Can you work these out from the model? Positions are in its coordinate system, mm. A direction names the side the tool comes from. Round coordinates to 2 decimals unless told otherwise and drop trailing zeros. Write each loop counter-clockwise with the first axis right and the second up, starting at its lowest first coordinate (ties: lowest second). Pieces come first, ordered by that corner, then holes. Notation, with made-up numbers: M -33,71 L 8,71 A22 cw 8,77 Z; hole C 38,-18 d1. An arc over 180 degrees is marked long. Answer in a Markdown table with one row per item. Add a question column.
(1) For faces 1 (the face through (76.2, -7, 9)), 2 (the face through (-76.2, -174, 85)), 3 (the face through (76.2, -151, -6)), 4 (the face through (-76.2, -7, 9)), which set-ups out of +Z, -Z, +X, -X, +Y, -Y let a thin tool reach every point of the face, with its end or its side?
(2) Suppose I cut it at D-D, the plane y = -191. Write out the boundary of the cut face in (x, z), then the cut area to 3 significant figures.
(3) Suppose I cut it at A-A, the plane z = 86.5. Write out the boundary of the cut face in (x, y).
(4) Suppose I cut it at C-C, the plane y = -152.5. Write out the boundary of the cut face in (x, z), then the cut area to 3 significant figures.
(5) If we mould it in two halves opening along X, with no side actions, what happens to faces 5 (the face through (-82.55, -174, 65)), 6 (the face through (76.2, -174, 85)), 7 (the face through (79, -50.8, 13)), 8 (the face through (64.74, 65.34, 9.66))? For each: released by +X, released by -X, zero draft, split by the parting line, or undercut.
(6) If I drill on probe 1 along Y at (x, z) = (0, 4.5); probe 2 along X at (y, z) = (-227.5, 41.5); probe 3 along Z at (x, y) = (-47, -205), over which ranges is the centre line in solid material (lowest first)?
(7) Suppose I cut it at B-B, the plane x = 0. Write out the boundary of the cut face in (y, z).
(8) I'm going to push flat-ended pins straight in: pin 1 (6 mm diameter, centred on x = 5, y = -165, fed in from +Z); pin 2 (9.5 mm diameter, centred on y = 6.5, z = 14, fed in from +X); pin 3 (9.5 mm diameter, centred on y = 5, z = 9, fed in from -X). Where does each tip first touch, or does it pass through?
from build123d import *

# Parameters (mm, degrees)
SKETCH2_W           = 152.4
SKETCH2_H           = 330.2
BOSS_EXTRUDE1_DEPTH = 19.05
SKETCH5_R           = 25.4
CUT_EXTRUDE1_DEPTH  = 266.867151976
FILLET1_R           = 38.1
BOSS_EXTRUDE2_DEPTH = 6.35


with BuildPart() as part:
    # Sketch2 → Boss-Extrude1 (new body)
    with BuildSketch(Plane.XY):
        with Locations((0, -88.9)):
            Rectangle(SKETCH2_W, SKETCH2_H)
    extrude(amount=BOSS_EXTRUDE1_DEPTH)

    # Sketch5 → Cut-Extrude1 (cut, through all)
    with BuildSketch(Plane.XY):
        with Locations(Location((0, 0, 0), (0, 0, 180))):
            Circle(SKETCH5_R)
    extrude(amount=CUT_EXTRUDE1_DEPTH, mode=Mode.SUBTRACT)

    # Fillet1
    fillet1_edges = [part.edges().sort_by_distance(p)[0] for p in [
        (-76.2, 76.2, 9.525),
        (76.2, 76.2, 9.525),
    ]]
    fillet(fillet1_edges, radius=FILLET1_R)

    # Sketch3 → Boss-Extrude2 (add)
    with BuildSketch(Plane(origin=(76.2, 0, 0), x_dir=(0, 0, -1), z_dir=(1, 0, 0))):
        Polygon((12.7, -50.8), (12.7, -254), (-190.5, -254), (-190.5, -203.2), (-38.1, -50.8), align=None)
    boss_extrude2 = extrude(amount=BOSS_EXTRUDE2_DEPTH)

    # Mirror1: Boss-Extrude2 across plane
    add(boss_extrude2.mirror(Plane(origin=(0, 0, 0), x_dir=(0, 0, 1), z_dir=(1, 0, 0))))


solid = part.part
Calculated:
| question | item | result |
|---|---|---|
| 1 | face 1 | +Z, -Z, +X, +Y |
| 1 | face 2 | +Z, +Y, -Y |
| 1 | face 3 | -Z, +Y, -Y |
| 1 | face 4 | +Z, -Z, -X, +Y |
| 2 | outline | M -82.55,-12.7 L -76.2,-12.7 L -76.2,0 L 76.2,0 L 76.2,-12.7 L 82.55,-12.7 L 82.55,178.3 L 76.2,178.3 L 76.2,19.05 L -76.2,19.05 L -76.2,178.3 L -82.55,178.3 Z |
| 2 | area | 5,330 mm² |
| 3 | outline | M -82.55,-254 L -76.2,-254 L -76.2,-99.2 L -82.55,-99.2 Z; M 76.2,-254 L 82.55,-254 L 82.55,-99.2 L 76.2,-99.2 Z |
| 4 | outline | M -82.55,-12.7 L -76.2,-12.7 L -76.2,0 L 76.2,0 L 76.2,-12.7 L 82.55,-12.7 L 82.55,139.8 L 76.2,139.8 L 76.2,19.05 L -76.2,19.05 L -76.2,139.8 L -82.55,139.8 Z |
| 4 | area | 4,840 mm² |
| 5 | face 5 | released by -X |
| 5 | face 6 | undercut |
| 5 | face 7 | zero draft |
| 5 | face 8 | released by +X |
| 6 | probe 1 | -254 to -25.4, 25.4 to 76.2 |
| 6 | probe 2 | -82.55 to -76.2, 76.2 to 82.55 |
| 6 | probe 3 | 0 to 19.05 |
| 7 | outline | M -254,0 L -25.4,0 L -25.4,19.05 L -254,19.05 Z; M 25.4,0 L 76.2,0 L 76.2,19.05 L 25.4,19.05 Z |
| 8 | pin 1 | z = 19.05 |
| 8 | pin 2 | x = 76.2 |
| 8 | pin 3 | x = -76.2 |
